from build123d import *

# Parameters (mm, degrees)
SKETCH1_R           = 30
BOSS_EXTRUDE1_DEPTH = 25
CUT_EXTRUDE1_DEPTH  = 5
CIRPATTERN1_COUNT   = 6
CUT_EXTRUDE2_START  = -10
SKETCH3_R           = 25
SKETCH3_R_2         = 10
SKETCH3_R_3         = 3
CUT_EXTRUDE2_DEPTH  = 10
BOSS_EXTRUDE2_START = 1
SKETCH4_R           = 30
SKETCH4_R_2         = 27.021684923
BOSS_EXTRUDE2_DEPTH = 1


with BuildPart() as part:
    # Sketch1 → Boss-Extrude1 (new body)
    with BuildSketch(Plane(origin=(0, 0, 0), x_dir=(0, 0, -1), z_dir=(1, 0, 0))):
        Circle(SKETCH1_R)
    extrude(amount=BOSS_EXTRUDE1_DEPTH)

    # Sketch2 → Cut-Extrude1 (cut)
    with BuildSketch(Plane.ZY):
        with BuildLine():
            Line((0, 25), (0, 5))
            ThreePointArc((0, 5), (1.225953008, 4.847374467), (2.377061324, 4.398815689))
            Line((2.377061324, 4.398815689), (4.016525549, 24.675241083))
            Line((4.016525549, 24.675241083), (0, 25))
        make_face()
        with BuildLine():
            ThreePointArc((-2.377061324, 4.398815689), (-1.225953008, 4.847374467), (0, 5))
            Line((0, 5), (0, 25))
            Line((0, 25), (-4.016525549, 24.675241083))
            Line((-4.016525549, 24.675241083), (-2.377061324, 4.398815689))
        make_face()
        with BuildLine():
            ThreePointArc((4.016525549, 24.675241083), (2.014816731, 24.918678005), (0, 25))
            Line((0, 25), (4.016525549, 24.675241083))
        make_face()
        with BuildLine():
            Line((-4.016525549, 24.675241083), (0, 25))
            ThreePointArc((0, 25), (-2.014816731, 24.918678005), (-4.016525549, 24.675241083))
        make_face()
    cut_extrude1 = extrude(amount=-CUT_EXTRUDE1_DEPTH, mode=Mode.SUBTRACT)

    # CirPattern1: Cut-Extrude1 ×6 about axis
    cirpattern1_axis = Axis((0, -0.752840444, 0), (1, 0, 0))
    for i in range(1, CIRPATTERN1_COUNT):
        add(cut_extrude1.rotate(cirpattern1_axis, i * 360 / CIRPATTERN1_COUNT), mode=Mode.SUBTRACT)

    # Sketch3 → Cut-Extrude2 (cut)
    # profile 1 of 2: a face of its own
    with BuildSketch(Plane(origin=(25, 0, 0), x_dir=(0, 0, -1), z_dir=(1, 0, 0)).offset(CUT_EXTRUDE2_START)):
        Circle(SKETCH3_R)
        Circle(SKETCH3_R_2, mode=Mode.SUBTRACT)
    # profile 2 of 2: a face of its own
    with BuildSketch(Plane(origin=(25, 0, 0), x_dir=(0, 0, -1), z_dir=(1, 0, 0)).offset(CUT_EXTRUDE2_START)):
        Circle(SKETCH3_R_3)
    extrude(amount=CUT_EXTRUDE2_DEPTH, mode=Mode.SUBTRACT)

    # Sketch4 → Boss-Extrude2 (add)
    with BuildSketch(Plane.ZY.offset(BOSS_EXTRUDE2_START)):
        Circle(SKETCH4_R)
        Circle(SKETCH4_R_2, mode=Mode.SUBTRACT)
    extrude(amount=-BOSS_EXTRUDE2_DEPTH)


solid = part.part
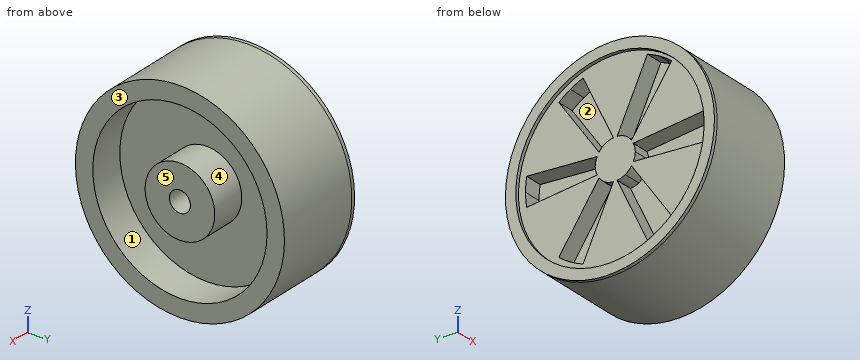
The model under review builds one solid part; all positions refer to its coordinate system, in mm. Face numbers are marked on the shaded views. A direction names the side the tool comes from. Coordinates: 2 decimals unless noted, no trailing zeros. Write each loop counter-clockwise with the first axis right and the second up, starting at its lowest first coordinate (ties: lowest second). Pieces come first, ordered by that corner, then holes. Notation, with made-up numbers: (47.5, 24.25) - (65.5, 24.25) arc R21 ccw to (65.5, 49.25) - close; hole circle Ø5 at (47.25, 37). An arc over 180 degrees is marked (long way). Answer as a JSON object with one key per item and string values. Group by question number.
1. Add section C-C (x = 3.5). Give the boundary of the cut face in (y, z).
2. Mouldability with a two-part tool opening along Z and no side actions: class the marked faces 4 and 5 as pulls with the +Z half, pulls with the -Z half, needs draft (parallel to the pull), parting line crosses it, or undercut.
3. Machinability: for the marked faces 1, 2 and 3, which of the approach directions +Z, -Z, +X, -X, +Y, -Y give a long, thin tool a straight path to every point of the face, cutting with its end or side? Answer none if there is none.
4. Add section D-D (x = 8.5). Give the boundary of the cut face in (y, z), plus the area to 3 significant figures.
5. Add section B-B (y = -20). Give the boundary of the cut face in (x, z).
6. Add section A-A (x = 22.5). Give the boundary of the cut face in (y, z), plus the area to 3 significant figures.
7. Clearance check with flat-ended pins moving along their axes: pin 1 Ø8 at (x, y) = (16.5, -17.5) entering from +Z; pin 2 Ø8 at (y, z) = (8.5, -10) entering from -X; pin 3 Ø5.5 at (y, z) = (0, 0) entering from +X; pin 4 Ø10 at (y, z) = (11, -6) entering from +X. State where each tip first meets the part, or that it passes through.
8. To check wall thickness, follow probe 1 along Y at (x, z) = (19.5, 0); probe 2 along Y at (x, z) = (21.75, -3.5); probe 3 along Z at (x, y) = (3.5, -9.5). State the ranges of each line that lie inside material, in increasing order.
Findings:
{
 "1": {"outline": "circle Ø60 at (0, 0); hole (-26.18, -4.02) - (-5.9, -2.38) arc R5 cw to (-5.9, 2.38) - (-26.18, 4.02) arc R25 ccw to start; hole (-16.95, -20.01) arc R25 ccw to (-9.99, -24.03) - (-1.27, -5.65) arc R5 cw to (-5.39, -3.27) - close; hole (-16.95, 20.01) - (-5.39, 3.27) arc R5 cw to (-1.27, 5.65) - (-9.99, 24.03) arc R25 ccw to start; hole (-0.24, -5.65) - (8.48, -24.03) arc R25 ccw to (15.44, -20.01) - (3.88, -3.27) arc R5 cw to start; hole (-0.24, 5.65) arc R5 cw to (3.88, 3.27) - (15.44, 20.01) arc R25 ccw to (8.48, 24.03) - close; hole (4.4, -2.38) - (24.68, -4.02) arc R25 ccw to (24.68, 4.02) - (4.4, 2.38) arc R5 cw to start"},
 "2": {"face 4": "undercut", "face 5": "needs draft"},
 "3": {"face 1": "+X", "face 2": "-X", "face 3": "+Z, -Z, +X, +Y, -Y"},
 "4": {"outline": "circle Ø60 at (0, 0)", "area": "2,830 mm²"},
 "5": {"outline": "(-1, -22.36) - (25, -22.36) - (25, -15) - (15, -15) - (15, 15) - (25, 15) - (25, 22.36) - (-1, 22.36) - (-1, 18.17) - (0, 18.17) - (0, 3.52) - (5, 3.52) - (5, -3.52) - (0, -3.52) - (0, -18.17) - (-1, -18.17) - close"},
 "6": {"outline": "circle Ø60 at (0, 0); circle Ø20 at (0, 0); hole circle Ø50 at (0, 0); hole circle Ø6 at (0, 0)", "area": "1,150 mm²"},
 "7": {"pin 1": "z = 26.79", "pin 2": "x = 0", "pin 3": "x = 15", "pin 4": "x = 25"},
 "8": {"probe 1": "-30 to -25, -10 to -3, 3 to 10, 25 to 30", "probe 2": "-29.8 to -24.75, -9.37 to 9.37, 24.75 to 29.8", "probe 3": "-28.46 to -23, -9.23 to -2.67, 2.67 to 9.23, 23 to 28.46"}
}
